For this review, take the finished solid that the model builds, in its own axes (mm). Face numbers are marked on the shaded views. A direction names the side the tool comes from. Coordinates: 2 decimals unless noted, no trailing zeros. Write each loop counter-clockwise with the first axis right and the second up, starting at its lowest first coordinate (ties: lowest second). Pieces come first, ordered by that corner, then holes.
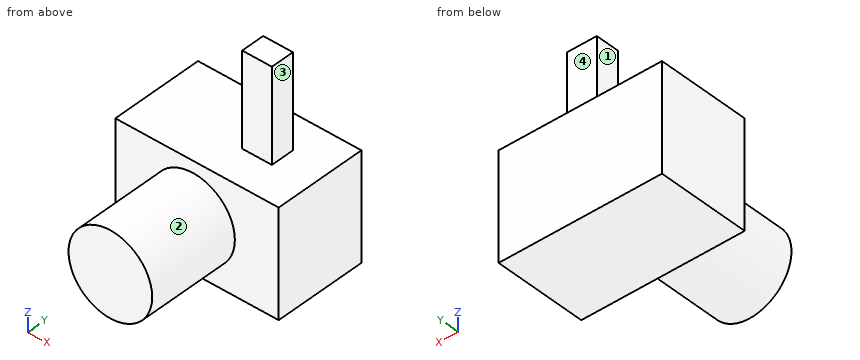
```python
from build123d import *

# Parameters (mm, degrees)
F0_W     = 44.574387
F0_H     = 29.136432
F1_DEPTH = 25.4
F2_W     = 8.096363
F2_H     = 6.445411
F3_DEPTH = 25.4
F4_R     = 11.414874
F5_DEPTH = 25.4


with BuildPart() as f1:
    # F0 (on Front) → F1 (new body)
    with BuildSketch(Plane.XZ):
        with Locations((-22.287194, 14.568216)):
            Rectangle(F0_W, F0_H)
    extrude(amount=F1_DEPTH)

    # F2 (on face) → F3 (join)
    with BuildSketch(Plane.XY.offset(29.136432)):
        with Locations((-14.480712, -12.520231)):
            Rectangle(F2_W, F2_H)
    extrude(amount=F3_DEPTH)

    # F4 (on face) → F5 (join)
    with BuildSketch(Plane.XZ.offset(25.4)):
        with Locations((-23.374369, 14.568217)):
            Circle(F4_R)
    extrude(amount=F5_DEPTH)


solid = f1.part
```
1) Consider section C-C (z = 37.5). Give the boundary of the cut face in (x, y).
2) Consider section D-D (x = -38.5). Give the boundary of the cut face in (y, z), then the cut area to 3 significant figures.
3) Clearance check with flat-ended pins moving along their axes: P1, Ø3, axis at x = -15.5, z = 45, coming from the +Y side; P2, Ø9, axis at x = -15.5, z = 38.5, coming from the -Y side; P3, Ø10, axis at x = -29.5, z = 36, coming from the -Y side; P4, Ø1.5, axis at x = -27, y = -38.5, coming from the +Z side. State where each tip first meets the part, or that it passes through.
4) For L1, parallel to Y at x = -4, z = 26; L2, parallel to Z at x = -25, y = -16; L3, parallel to X at y = -27, z = 15, list the stretches that pass through material, from the lowest coordinate up.
5) Tool access review of the marked faces 1, 2, 3 and 4: name each direction out of +Z, -Z, +X, -X, +Y, -Y from which nothing blocks a thin tool from reaching the whole face with its end or side.
6) Consider section A-A (y = -10). Give the boundary of the cut face in (x, z), then the cut area to 3 significant figures.
7) Consider section B-B (x = -34). Give the boundary of the cut face in (y, z), then the cut area to 3 significant figures.
Results:
1. outline: (-18.53, -15.74) - (-10.43, -15.74) - (-10.43, -9.3) - (-18.53, -9.3) - close
2. outline: (-25.4, 0) - (0, 0) - (0, 29.14) - (-25.4, 29.14) - close
2. area: 740 mm2
3. P1: stops at y = -9.3
3. P2: stops at y = -15.74
3. P3: passes through
3. P4: stops at z = 25.61
4. L1: y = -25.4 to 0
4. L2: z = 0 to 29.14
4. L3: x = -34.78 to -11.97
5. face 1: +Z, -X, +Y, -Y
5. face 2: -Y
5. face 3: +Z, +X, +Y, -Y
5. face 4: +Z, +X, -X, +Y
6. outline: (-44.57, 0) - (0, 0) - (0, 29.14) - (-10.43, 29.14) - (-10.43, 54.54) - (-18.53, 54.54) - (-18.53, 29.14) - (-44.57, 29.14) - close
6. area: 1,500 mm2
7. outline: (-50.8, 10.4) - (-25.4, 10.4) - (-25.4, 0) - (0, 0) - (0, 29.14) - (-25.4, 29.14) - (-25.4, 18.74) - (-50.8, 18.74) - close
7. area: 952 mm2
